The listing builds one solid part. Answer for the finished solid, in the listing's coordinates (mm). A direction names the side the tool comes from. Round coordinates to 2 decimals unless told otherwise and drop trailing zeros. Order: outer loops, then holes, each group sorted by start corner. A loop starts at its lowest first (then second) coordinate and runs counter-clockwise, first axis right, second up. Notation, with made-up numbers: (58.25, -7.5) -> (111.25, -7.5) arc R18 ccw to (111.25, 25.5) -> close; hole circle Ø1 at (80.5, -5.5). An arc over 180 degrees is marked (long way). Return JSON: item names as keys, results as strings. Group by question number.
(1) Determine the mould class of faces 1 (the face through (65, 20, -18)), 2 (the face through (72, 3, -1)), 3 (the face through (65.986, 21.003, -18.797)), 4 (the face through (-76.14, 1.52, -37.1)) for opening direction Z: +Z half, -Z half, draft (parallel to the pull), parting line (faces both ways), or undercut.
(2) The part is cut by section C-C (x = 44). Determine the outline of the cut face in (y, z).
(3) Each of these flat-tipped pins is pushed along its axis until it touches: pin 1 (3.5 mm diameter, centred on x = 72, z = 24.57, fed in from -Y); pin 2 (3 mm diameter, centred on y = 8.5, z = -3, fed in from +X); pin 3 (2 mm diameter, centred on y = 9, z = -26, fed in from -X); pin 4 (4 mm diameter, centred on x = 0.5, z = 13, fed in from +Y). Where does it stop, or does it pass through?
(4) The part is cut by section A-A (x = -72). Determine the outline of the cut face in (y, z).
(5) Consider line 1 (Z direction, x = 72, y = 2.1); line 2 (Z direction, x = -59, y = 8.5); line 3 (X direction, y = 21.5, z = 23). Determine where each line is inside the solid, lowest interval first. Write a range as [from, to].
(6) Which of the six approach directions +Z, -Z, +X, -X, +Y, -Y give full straight-line access (tool end or side, diameter ignored) to faces 5 (the face through (-67, 20, 1)), 6 (the face through (-1, 24, 38)), 7 (the face through (-65, 20, -18))?
(7) The part is cut by section B-B (y = 42). Determine the outline of the cut face in (x, z), plus the area to 3 significant figures.
(8) The part is cut by section D-D (y = 7). Determine the outline of the cut face in (x, z).
from build123d import *

# Parameters (mm, degrees)
SZKIC1_W                    = 154
SZKIC1_H                    = 76
DODANIE_WYCI_GNI_CIE1_DEPTH = 3
SZKIC1_3_W                  = 134
SZKIC1_3_H                  = 76
SZKIC1_3_W_2                = 130
SZKIC1_3_H_2                = 72
SZKIC1_3_H_3                = 2
DODANIE_WYCI_GNI_CIE2_DEPTH = 48
WYTNIJ_WYCI_GNI_CIE1_DEPTH  = 157.473639953
M3_CLEARANCE_HOLE1_D        = 3.2
M3_CLEARANCE_HOLE1_DEPTH    = 7.7
M3_CLEARANCE_HOLE1_TIP      = 0.96137699
ZAOKR_GLENIE1_R             = 3
SZKIC6_W                    = 21
SZKIC6_H                    = 2
WYTNIJ_WYCI_GNI_CIE2_DEPTH  = 119.359621493
SFAZOWANIE1_SIZE            = 1


with BuildPart() as part:
    # Szkic1 → Dodanie-wyciągnięcie1 (new body)
    with BuildSketch(Plane(origin=(0, 0, 0), x_dir=(1, 0, 0), z_dir=(0, 1, 0))):
        Rectangle(SZKIC1_W, SZKIC1_H)
    extrude(amount=DODANIE_WYCI_GNI_CIE1_DEPTH)

    # Szkic1<3> → Dodanie-wyciągnięcie2 (add)
    # profile 1 of 2: a face of its own
    with BuildSketch(Plane(origin=(0, 0, 0), x_dir=(1, 0, 0), z_dir=(0, 1, 0))):
        Rectangle(SZKIC1_3_W, SZKIC1_3_H)
        Rectangle(SZKIC1_3_W_2, SZKIC1_3_H_2, mode=Mode.SUBTRACT)
    # profile 2 of 2: a face of its own
    with BuildSketch(Plane(origin=(0, 0, 0), x_dir=(1, 0, 0), z_dir=(0, 1, 0))):
        Rectangle(SZKIC1_3_W_2, SZKIC1_3_H_3)
    extrude(amount=DODANIE_WYCI_GNI_CIE2_DEPTH)

    # Szkic2 → Wytnij-wyciągnięcie1 (cut, through all)
    with BuildSketch(Plane.ZY.offset(67)):
        with BuildLine():
            ThreePointArc((-5, 34.5), (-8.954058454, 44.045941546), (-18.5, 48))
            ThreePointArc((-18.5, 48), (-28.045941546, 44.045941546), (-32, 34.5))
            Line((-32, 34.5), (-5, 34.5))
        make_face()
        with BuildLine():
            Line((-5, 34.5), (-32, 34.5))
            ThreePointArc((-32, 34.5), (-18.5, 21), (-5, 34.5))
        make_face()
        with BuildLine():
            Line((-18.5, 48), (-32, 48))
            Line((-32, 48), (-32, 34.5))
            ThreePointArc((-32, 34.5), (-28.045941546, 44.045941546), (-18.5, 48))
        make_face()
        with BuildLine():
            Line((-5, 48), (-18.5, 48))
            ThreePointArc((-18.5, 48), (-8.954058454, 44.045941546), (-5, 34.5))
            Line((-5, 34.5), (-5, 48))
        make_face()
        with BuildLine():
            ThreePointArc((18.5, 48), (8.954058454, 44.045941546), (5, 34.5))
            Line((5, 34.5), (32, 34.5))
            ThreePointArc((32, 34.5), (28.045941546, 44.045941546), (18.5, 48))
        make_face()
        with BuildLine():
            Line((32, 34.5), (5, 34.5))
            ThreePointArc((5, 34.5), (18.5, 21), (32, 34.5))
        make_face()
        with BuildLine():
            Line((18.5, 48), (5, 48))
            Line((5, 48), (5, 34.5))
            ThreePointArc((5, 34.5), (8.954058454, 44.045941546), (18.5, 48))
        make_face()
        with BuildLine():
            Line((32, 48), (18.5, 48))
            ThreePointArc((18.5, 48), (28.045941546, 44.045941546), (32, 34.5))
            Line((32, 34.5), (32, 48))
        make_face()
    extrude(amount=-WYTNIJ_WYCI_GNI_CIE1_DEPTH, mode=Mode.SUBTRACT)

    # M3 Clearance Hole1
    with Locations(Plane(origin=(0, 3, 0), x_dir=(1, 0, 0), z_dir=(0, 1, 0))):
        with Locations((-72, 24.565309611), (-72, -24.565309611), (72, -24.565309611), (72, 24.565309611)):
            Hole(M3_CLEARANCE_HOLE1_D / 2, depth=M3_CLEARANCE_HOLE1_DEPTH)
            with Locations((0, 0, -(M3_CLEARANCE_HOLE1_DEPTH + M3_CLEARANCE_HOLE1_TIP / 2))):  # 118° drill point
                Cone(0, M3_CLEARANCE_HOLE1_D / 2, M3_CLEARANCE_HOLE1_TIP, mode=Mode.SUBTRACT)

    # Zaokrąglenie1
    zaokr_glenie1_edges = [part.edges().sort_by_distance(p)[0] for p in [
        (77, 1.5, 38),
        (77, 1.5, -38),
        (-77, 1.5, 38),
        (-77, 1.5, -38),
    ]]
    fillet(zaokr_glenie1_edges, radius=ZAOKR_GLENIE1_R)

    # Szkic6 → Wytnij-wyciągnięcie2 (cut, through all)
    with BuildSketch(Plane.XY.offset(38)):
        with Locations((0, 45)):
            Rectangle(SZKIC6_W, SZKIC6_H)
    extrude(amount=-WYTNIJ_WYCI_GNI_CIE2_DEPTH, mode=Mode.SUBTRACT)

    # Sfazowanie1
    sfazowanie1_edges = [part.edges().sort_by_distance(p)[0] for p in [
        (10.5, 44, 37),
        (10.5, 46, 37),
        (-10.5, 46, 37),
        (-10.5, 44, 37),
        (10.5, 46, -37),
        (10.5, 44, -37),
        (-10.5, 46, -37),
        (-10.5, 44, -37),
        (-10.5, 46, 0),
        (-10.5, 44, 0),
        (10.5, 46, 0),
        (10.5, 44, 0),
    ]]
    chamfer(sfazowanie1_edges, length=SFAZOWANIE1_SIZE - 0.0001)  # a hair under: the kernel refuses the full size


solid = part.part
Answer below:
{
 "1": {"face 1": "undercut", "face 2": "draft", "face 3": "undercut", "face 4": "-Z half"},
 "2": {"outline": "(0, -38) -> (48, -38) -> (48, -36) -> (3, -36) -> (3, -1) -> (48, -1) -> (48, 1) -> (3, 1) -> (3, 36) -> (48, 36) -> (48, 38) -> (0, 38) -> close"},
 "3": {"pin 1": "stops at y = 0", "pin 2": "stops at x = 67", "pin 3": "stops at x = -67", "pin 4": "stops at y = 3"},
 "4": {"outline": "(0, -38) -> (3, -38) -> (3, -26.17) -> (0, -26.17) -> close; (0, -22.97) -> (3, -22.97) -> (3, 22.97) -> (0, 22.97) -> close; (0, 26.17) -> (3, 26.17) -> (3, 38) -> (0, 38) -> close"},
 "5": {"line 1": "z = [-38, -26.17], [-22.97, 22.97], [26.17, 38]", "line 2": "z = [-38, -36], [-1, 1], [36, 38]", "line 3": "x = [-67, -65], [65, 67]"},
 "6": {"face 5": "+Z, -Z, -X, +Y", "face 6": "+Z, +X, -X, +Y, -Y", "face 7": "+Y"},
 "7": {"outline": "(-67, -38) -> (67, -38) -> (67, -32) -> (65, -32) -> (65, -36) -> (-65, -36) -> (-65, -32) -> (-67, -32) -> close; (-67, -5) -> (-65, -5) -> (-65, -1) -> (65, -1) -> (65, -5) -> (67, -5) -> (67, 5) -> (65, 5) -> (65, 1) -> (-65, 1) -> (-65, 5) -> (-67, 5) -> close; (-67, 32) -> (-65, 32) -> (-65, 36) -> (65, 36) -> (65, 32) -> (67, 32) -> (67, 38) -> (-67, 38) -> close", "area": "868 mm²"},
 "8": {"outline": "(-67, -38) -> (67, -38) -> (67, 38) -> (-67, 38) -> close; hole (-65, -36) -> (65, -36) -> (65, -1) -> (-65, -1) -> close; hole (-65, 1) -> (65, 1) -> (65, 36) -> (-65, 36) -> close"}
}
